Drawing for the job (mm, zero at the part's lowest x, y, z). A direction names the side the tool comes from. Round coordinates to 2 decimals unless told otherwise and drop trailing zeros. Loops run counter-clockwise (first coordinate to the right, second up) from the corner with the lowest first, then second, coordinate; pieces in that order, holes last.
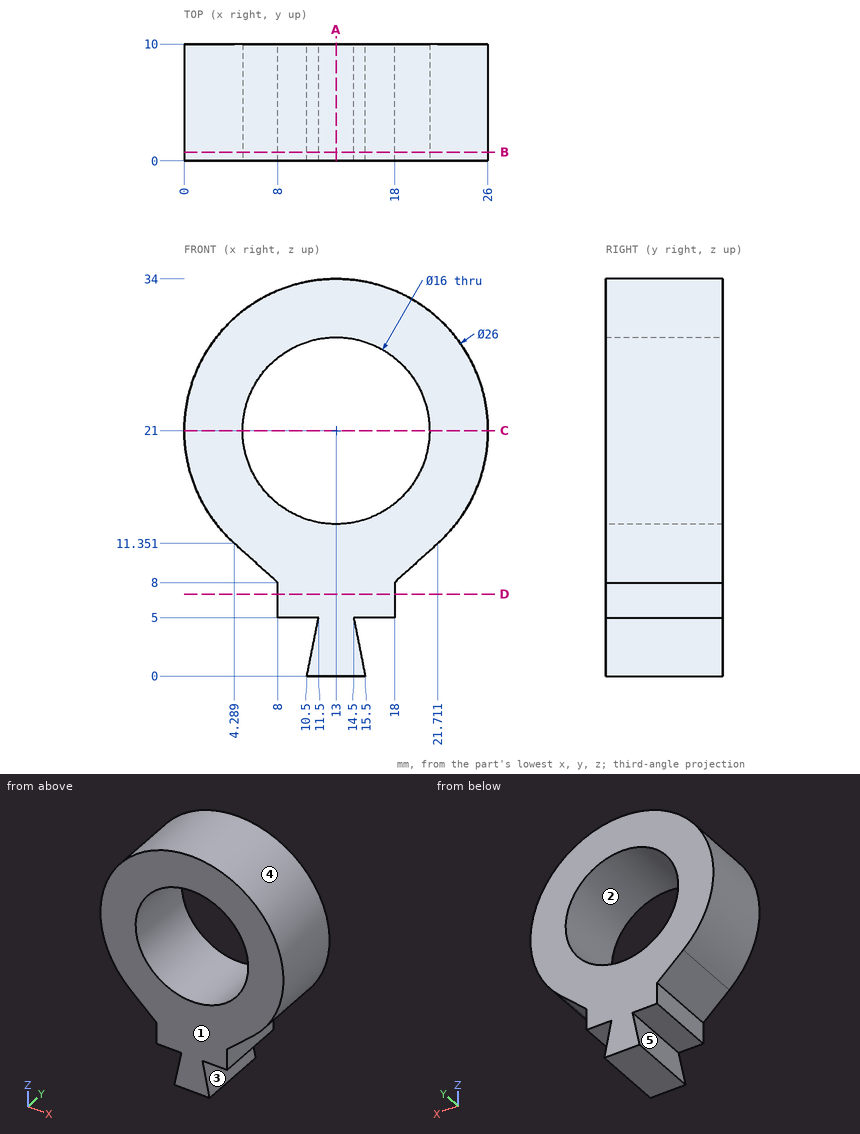
Q1. Probe line 1 (X direction, y = 6, z = 21); line 2 (X direction, y = 9, z = 7); line 3 (Z direction, x = 15.75, y = 8.75) (1 decimal). List the from-to ranges inside material, lowest first.
Q2. Flat gauge pins, fed straight in: P1, Ø1.5, axis at y = 6, z = 7, coming from the +X side; P2, Ø1.5, axis at y = 8.5, z = 17, coming from the +X side; P3, Ø2, axis at x = 20, y = 2, coming from the -Z side. Where does each tip first touch, or does it go through?
Q3. Slice it at D-D on z = 7. Give the cut face in (x, y), plus the area to 3 significant figures.
Q4. Slice it at C-C on z = 21. Give the cut face in (x, y), plus the area to 3 significant figures.
Q5. Slice it at B-B on y = 0.75. Give the cut face in (x, z), plus the area to 3 significant figures.
Q6. Slice it at A-A on x = 13. Give the cut face in (y, z).
Q7. Pull direction X, two halves, no side cores. Call the marked faces 1, 2 and 3: pulls with the +X half, pulls with the -X half, needs draft (parallel to the pull), parting line crosses it, or undercut.
Q8. Tool access for the marked faces 4 and 5: list every direction of +Z, -Z, +X, -X, +Y, -Y with a clear straight run to the whole face (end or side of a thin tool).
Reply:
1. line 1: x = 0 to 5, 21 to 26
1. line 2: x = 8 to 18
1. line 3: z = 5 to 13.5, 28.5 to 33.7
2. P1: stops at x = 18
2. P2: stops at x = 25.59
2. P3: stops at z = 8.9
3. outline: (8, 0) - (18, 0) - (18, 10) - (8, 10) - close
3. area: 100 mm2
4. outline: (0, 0) - (5, 0) - (5, 10) - (0, 10) - close; (21, 0) - (26, 0) - (26, 10) - (21, 10) - close
4. area: 100 mm2
5. outline: (4.29, 11.35) - (8, 8) - (8, 5) - (11.5, 5) - (10.5, 0) - (15.5, 0) - (14.5, 5) - (18, 5) - (18, 8) - (21.71, 11.35) arc R13 ccw (long way) to start; hole circle Ø16 at (13, 21)
5. area: 386 mm2
6. outline: (0, 0) - (10, 0) - (10, 13) - (0, 13) - close; (0, 29) - (10, 29) - (10, 34) - (0, 34) - close
7. face 1: needs draft
7. face 2: undercut
7. face 3: pulls with the +X half
8. face 4: +Y, -Y
8. face 5: -X, +Y, -Y
